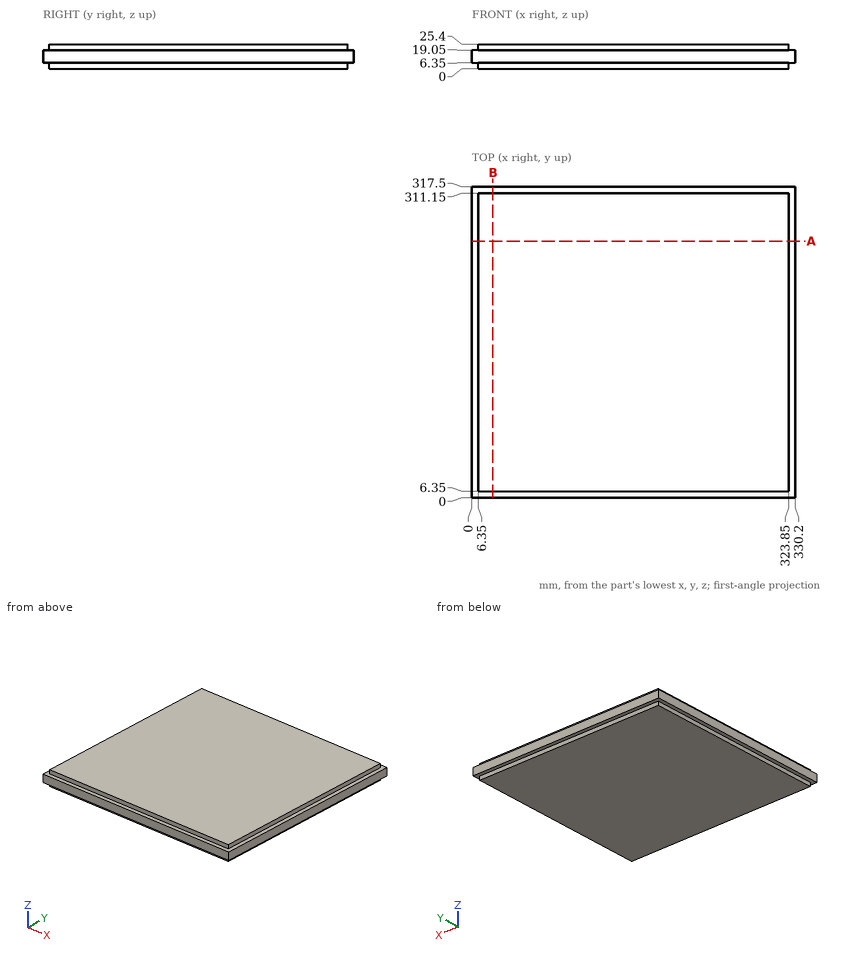
Input: dimensioned drawing with shaded views. Units: mm. Origin: part minimum x, y, z. Give positions to 0.01 mm unless a question says otherwise; leave off trailing zeros. Write each loop counter-clockwise with the first axis right and the second up, starting at its lowest first coordinate (ties: lowest second). Pieces come first, ordered by that corner, then holes. Notation, with made-up numbers: (63.5, 52) -> (90.5, 52) arc R15 cw to (90.5, 76) -> close; hole circle Ø9 at (82.25, 27.5). An arc over 180 degrees is marked (long way). Return JSON: item names as keys, results as strings. Group by question number.
1. Material intervals for line 1 (X direction, y = 154, z = 1.5); line 2 (Y direction, x = 133, z = 2), sorted ascending. Write a range as from..to.
2. Section B-B, the plane x = 21.5. Output: boundary loops of the cut face in (y, z), then the cut area to 3 significant figures.
3. Section A-A, the plane y = 262. Output: boundary loops of the cut face in (x, z), then the cut area to 3 significant figures.
4. Pin query (flat end, axial travel): pin 1 Ø1.9 at (x, z) = (167, 4.5) entering from +Y; pin 2 Ø3 at (x, z) = (132, 21.5) entering from -Y; pin 3 Ø7 at (y, z) = (225.5, 23.5) entering from +X. Return the tip coordinate at first contact, or that it passes through.
Determined:
{
 "1": {"line 1": "x = 6.35..323.85", "line 2": "y = 6.35..311.15"},
 "2": {"outline": "(0, 6.35) -> (6.35, 6.35) -> (6.35, 0) -> (311.15, 0) -> (311.15, 6.35) -> (317.5, 6.35) -> (317.5, 19.05) -> (311.15, 19.05) -> (311.15, 25.4) -> (6.35, 25.4) -> (6.35, 19.05) -> (0, 19.05) -> close", "area": "7,900 mm2"},
 "3": {"outline": "(0, 6.35) -> (6.35, 6.35) -> (6.35, 0) -> (323.85, 0) -> (323.85, 6.35) -> (330.2, 6.35) -> (330.2, 19.05) -> (323.85, 19.05) -> (323.85, 25.4) -> (6.35, 25.4) -> (6.35, 19.05) -> (0, 19.05) -> close", "area": "8,230 mm2"},
 "4": {"pin 1": "stops at y = 311.15", "pin 2": "stops at y = 6.35", "pin 3": "stops at x = 323.85"}
}
